The figure shows three views and two pictorial views of one solid part (mm, origin at its lowest corner). Answer the questions. Coordinates: 2 decimals unless noted, no trailing zeros. Order: outer loops, then holes, each group sorted by start corner. A loop starts at its lowest first (then second) coordinate and runs counter-clockwise, first axis right, second up. Notation, with made-up numbers: (83.25, 11.25) -> (89.25, 11.25) arc R15 ccw to (89.25, 18.25) -> close; hole circle Ø10 at (7.25, 35). An arc over 180 degrees is marked (long way). Return JSON: item names as keys, results as strings.
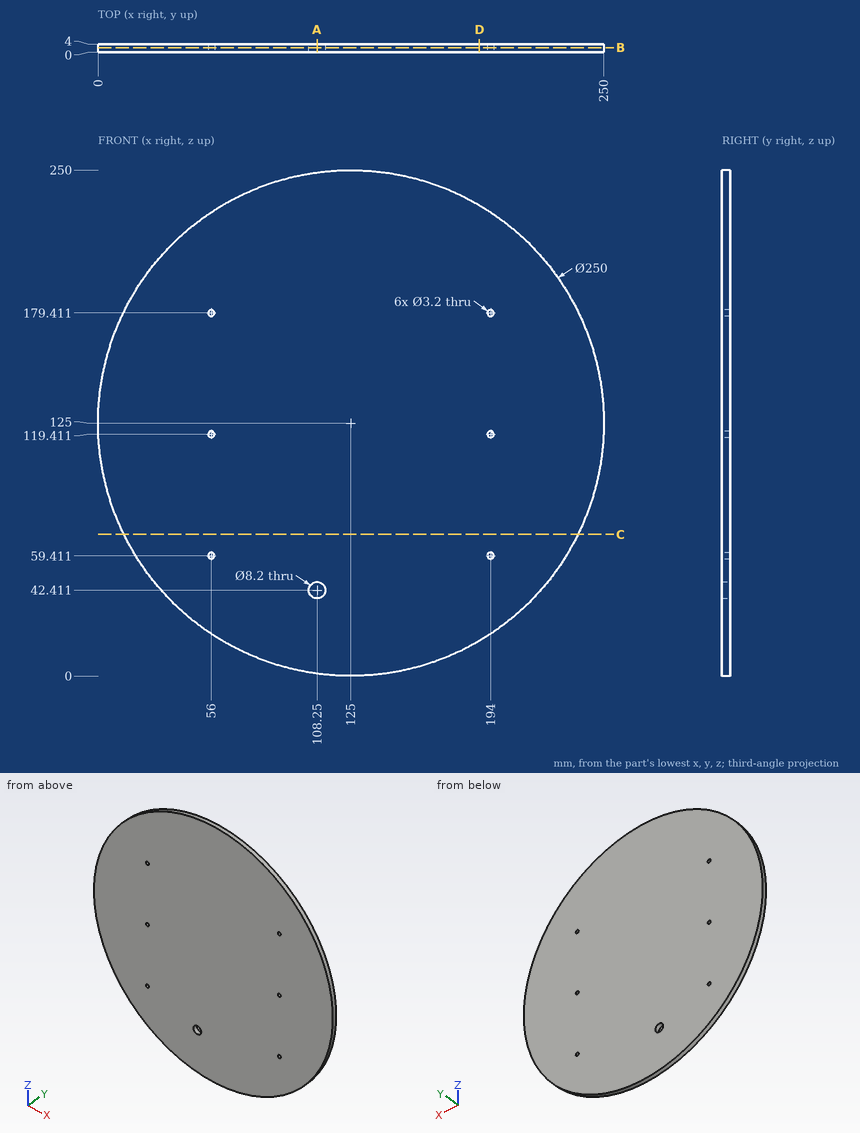
1. The part is cut by section A-A on x = 108.25. Give the vertices of the cut face in (y, z).
Answer block:
{"outline": "(0, 1.13) -> (4, 1.13) -> (4, 38.31) -> (0, 38.31) -> close; (0, 46.51) -> (4, 46.51) -> (4, 248.87) -> (0, 248.87) -> close"}
2. Each of these flat-tipped pins is pushed along its axis until it touches: pin 1 Ø9.5 at (x, z) = (108.25, 42.411) entering from -Y; pin 2 Ø2 at (x, y) = (37, 0.5) entering from -Z; pin 3 Ø1 at (y, z) = (0.5, 193.5) entering from +X. Where does it stop, or does it pass through?
Answer block:
{"pin 1": "stops at y = 0", "pin 2": "stops at z = 35.24", "pin 3": "stops at x = 229.89"}
3. Consider line 1 (Z direction, x = 56, y = 2.6); line 2 (X direction, y = 2.85, z = 39); line 3 (Z direction, x = 108.25, y = 1.9). Determine where each line is inside the solid, lowest interval first. Write a range as from..to.
Answer block:
{"line 1": "z = 20.77..57.81, 61.01..117.81, 121.01..177.81, 181.01..229.23", "line 2": "x = 34.29..105.98, 110.52..215.71", "line 3": "z = 1.13..38.31, 46.51..248.87"}
4. The part is cut by section D-D on x = 188.5. Give the vertices of the cut face in (y, z).
Answer block:
{"outline": "(0, 17.33) -> (4, 17.33) -> (4, 232.67) -> (0, 232.67) -> close"}
5. The part is cut by section C-C on z = 70. Give the vertices of the cut face in (x, y), and give its area (3 significant figures).
Answer block:
{"outline": "(12.75, 0) -> (237.25, 0) -> (237.25, 4) -> (12.75, 4) -> close", "area": "898 mm2"}
6. The part is cut by section B-B on y = 2.2. Give the vertices of the cut face in (x, z), and give its area (3 significant figures).
Answer block:
{"outline": "circle Ø250 at (125, 125); hole circle Ø3.2 at (56, 59.41); hole circle Ø3.2 at (56, 119.41); hole circle Ø3.2 at (56, 179.41); hole circle Ø8.2 at (108.25, 42.41); hole circle Ø3.2 at (194, 59.41); hole circle Ø3.2 at (194, 119.41); hole circle Ø3.2 at (194, 179.41)", "area": "49,000 mm2"}
